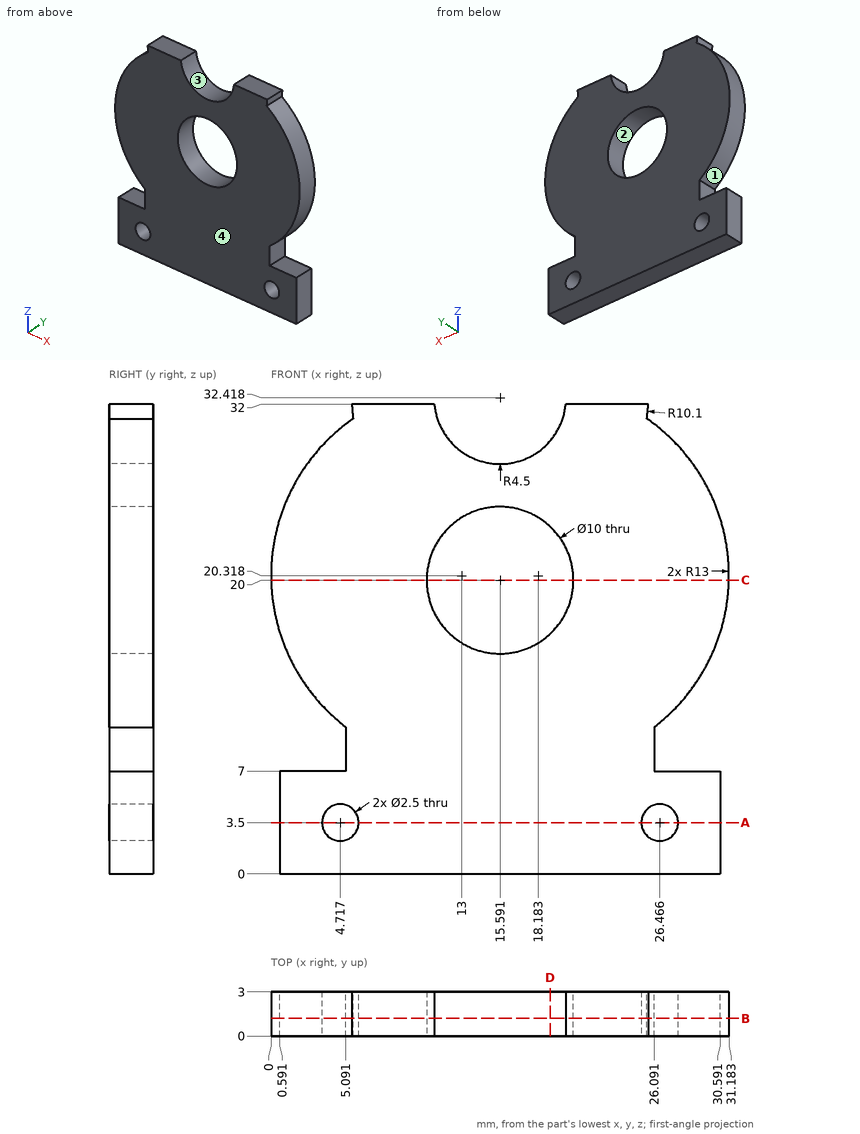
For this review, use the dimensioned drawing (mm, ordinates from the lowest corner) and the shaded views. Coordinates: 2 decimals unless noted, no trailing zeros. Write each loop counter-clockwise with the first axis right and the second up, starting at its lowest first coordinate (ties: lowest second). Pieces come first, ordered by that corner, then holes. Notation, with made-up numbers: (8.25, -3.75) - (29.25, -3.75) arc R29 cw to (29.25, 24.25) - close; hole circle Ø11 at (33.25, -16). An arc over 180 degrees is marked (long way). Answer as a JSON object with one key per item and string values. Group by question number.
1. Add section D-D (x = 19). Give the boundary of the cut face in (y, z).
2. Clearance check with flat-ended pins moving along their axes: pin 1 Ø0.9 at (y, z) = (1.5, 9) entering from +X; pin 2 Ø1 at (x, y) = (16.5, 2.5) entering from +Z; pin 3 Ø1.5 at (y, z) = (1.5, 8.5) entering from -X; pin 4 Ø1 at (x, y) = (18, 0.5) entering from -Z. State where each tip first meets the part, or that it passes through.
3. Add section C-C (z = 20). Give the boundary of the cut face in (x, y).
4. Mouldability with a two-part tool opening along X and no side actions: class the marked faces 1, 2, 3 and 4 as pulls with the +X half, pulls with the -X half, needs draft (parallel to the pull), parting line crosses it, or undercut.
5. To check wall thickness, follow probe 1 along X at (y, z) = (2.2, 17); probe 2 along X at (y, z) = (2.8, 30) (1 decimal); probe 3 along X at (y, z) = (1.8, 4.5) (1 decimal). State the ranges of each line that lie inside material, in increasing order.
6. Add section B-B (y = 1.2). Give the boundary of the cut face in (x, z).
7. Add section A-A (z = 3.5). Give the boundary of the cut face in (x, y).
Findings:
{
 "1": {"outline": "(0, 0) - (3, 0) - (3, 16.34) - (0, 16.34) - close; (0, 23.66) - (3, 23.66) - (3, 29.48) - (0, 29.48) - close"},
 "2": {"pin 1": "x = 26.09", "pin 2": "z = 28.14", "pin 3": "x = 5.09", "pin 4": "z = 0"},
 "3": {"outline": "(0, 0) - (10.59, 0) - (10.59, 3) - (0, 3) - close; (20.59, 0) - (31.18, 0) - (31.18, 3) - (20.59, 3) - close"},
 "4": {"face 1": "pulls with the -X half", "face 2": "undercut", "face 3": "undercut", "face 4": "needs draft"},
 "5": {"probe 1": "0.43 to 11.59, 19.59 to 30.75", "probe 2": "4.3 to 11.8, 19.4 to 26.9", "probe 3": "0.6 to 4, 5.5 to 25.7, 27.2 to 30.6"},
 "6": {"outline": "(0.59, 0) - (30.59, 0) - (30.59, 7) - (26.09, 7) - (26.09, 10) arc R13 ccw to (25.59, 31) arc R10.1 ccw to (25.68, 32) - (20.07, 32) arc R4.5 cw to (11.11, 32) - (5.5, 32) arc R10.1 ccw to (5.59, 31) arc R13 ccw to (5.09, 10) - (5.09, 7) - (0.59, 7) - close; hole circle Ø2.5 at (4.72, 3.5); hole circle Ø10 at (15.59, 20); hole circle Ø2.5 at (26.47, 3.5)"},
 "7": {"outline": "(0.59, 0) - (3.47, 0) - (3.47, 3) - (0.59, 3) - close; (5.97, 0) - (25.22, 0) - (25.22, 3) - (5.97, 3) - close; (27.72, 0) - (30.59, 0) - (30.59, 3) - (27.72, 3) - close"}
}
